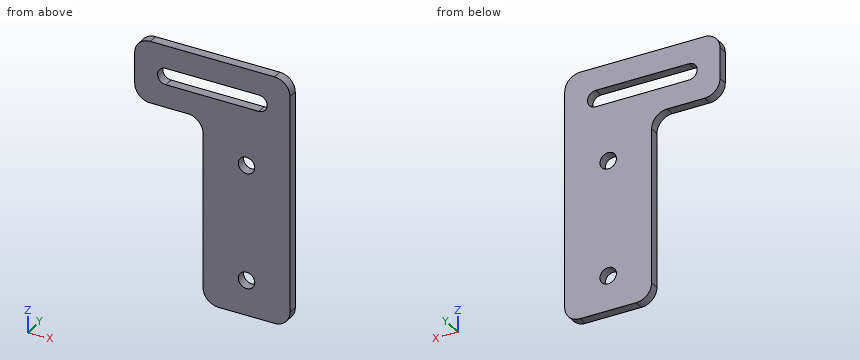
Autodesk Inventor part; units mm, degrees
ref_plane "YZ Plane" through (0, 0, 0) normal (1, 0, 0) x (0, 1, 0)
ref_plane "XZ Plane" through (0, 0, 0) normal (0, 1, 0) x (-1, 0, 0)
ref_plane "XY Plane" through (0, 0, 0) normal (0, 0, 1) x (1, 0, 0)
sketch "Sketch1" plane through (0, 0, 0) normal (0, 1, 0) x (-1, 0, 0)
  line L0 (-25, 40) -> (25, 40)
  line L1 (25, 40) -> (25, -40)
  line L2 (25, -40) -> (-25, -40)
  line L3 (-25, -40) -> (-25, 40)
  line L4 (-25, 40) -> (25, -40) construction
  line L5 (25, 40) -> (-25, -40) construction
  point P0 (0, 0)
  dimension "d0" = 50
  dimension "d1" = 80
extrude "Extrusion1" add sketch "Sketch1" along normal blind 3
sketch "Sketch2" plane through (0, 3, 0) normal (0, 1, 0) x (1, 0, 0)
  line L0 (25, -40) -> (25, 40)
  line L1 (25, 40) -> (11, 40)
  line L2 (11, 40) -> (11, 28.65)
  line L3 (11, 28.65) -> (25, 28.65)
  line L4 (25, 28.65) -> (25, 40)
  line L5 (11, 28.65) -> (11, -8.65)
  circle A0 centre (11, 28.65) radius 2.65
  circle A1 centre (11, -8.65) radius 2.65
  line L6 (-25, -40) -> (25, -40)
  line L7 (-25, 40) -> (-25, -40)
  line L8 (25, -40) -> (-25, -40)
  line L9 (-25, -40) -> (-25, -30)
  line L10 (-25, -30) -> (25, -30)
  line L11 (25, -30) -> (25, -40)
  line L12 (25, -30) -> (15, -30)
  line L13 (-25, -30) -> (-15, -30)
  line L14 (-15, -30) -> (15, -30) construction
  line L15 (-15, -32.65) -> (15, -32.65)
  line L16 (15, -27.35) -> (-15, -27.35)
  arc A2 (-15, -27.35) -> (-15, -32.65) centre (-15, -30) ccw
  arc A3 (15, -32.65) -> (15, -27.35) centre (15, -30) ccw
  line L17 (-25, -30) -> (-25, 40)
  line L18 (-25, 40) -> (-3, 40)
  line L19 (-3, 40) -> (-3, -20)
  line L20 (-3, -20) -> (-25, -20)
  point P0 (0, 0)
  point P1 (0, -30)
  dimension "d4" = 14
  dimension "d5" = 11.35
  dimension "d6" = 37.3
  dimension "d7" = 5.3
  dimension "d8" = 5.3
  dimension "d9" = 10
  dimension "d10" = 10
  dimension "d11" = 10
  dimension "d12" = 5.3
  dimension "d13" = 22
  dimension "d14" = 60
extrude "Extrusion2" cut sketch "Sketch2" against normal through all contours L7 L18 L19 L20 | A1 | A3 L15 A2 L10 | L10 A2 L16 A3 | A0 L5 L3 | L3 L2 A0 | L5 A0 L2
fillet "Fillet1" radius 5 6 edges at (-25, 1.5, 40) (25, 1.5, 40) (25, 1.5, -40) (-3, 1.5, -40) (-3, 1.5, 20) (-25, 1.5, 20)
properties part number "LeadScrewEndMount"
Verification items for the finished model (mm, model axes). Round coordinates to 2 decimals unless told otherwise and drop trailing zeros. Write each loop counter-clockwise with the first axis right and the second up, starting at its lowest first coordinate (ties: lowest second). Pieces come first, ordered by that corner, then holes.
1. Section check C-C on y = 2. Enter the section's corners in (x, z), plus the area to 3 significant figures.
2. Section check A-A on x = 11. Enter the section's corners in (y, z), plus the area to 3 significant figures.
3. Scan lines: L1, parallel to Z at x = 11, y = 0.95; L2, parallel to X at y = 1.8, z = -28.65; L3, parallel to X at y = 2.8, z = -23.5. Record each from-to range of solid material in increasing order.
4. Section check D-D on x = 16. Enter the section's corners in (y, z), plus the area to 3 significant figures.
5. Gauge pin test, flat ends, axial feed: P1, Ø1.5, axis at y = 1, z = -6.5, coming from the -X side; P2, Ø3, axis at x = 11, z = 8.65, coming from the +Y side. Record the tip position at first contact, or that the pin passes through.
6. Section check B-B on z = -28.65. Enter the section's corners in (x, y), plus the area to 3 significant figures.
Answer:
1. outline: (-25, 25) arc R5 ccw to (-20, 20) - (-8, 20) arc R5 cw to (-3, 15) - (-3, -35) arc R5 ccw to (2, -40) - (20, -40) arc R5 ccw to (25, -35) - (25, 35) arc R5 ccw to (20, 40) - (-20, 40) arc R5 ccw to (-25, 35) - close; hole (-15, 27.35) - (15, 27.35) arc R2.65 ccw to (15, 32.65) - (-15, 32.65) arc R2.65 ccw to start; hole circle Ø5.3 at (11, -28.65); hole circle Ø5.3 at (11, 8.65)
1. area: 2,430 mm2
2. outline: (0, -40) - (3, -40) - (3, -31.3) - (0, -31.3) - close; (0, -26) - (3, -26) - (3, 6) - (0, 6) - close; (0, 11.3) - (3, 11.3) - (3, 27.35) - (0, 27.35) - close; (0, 32.65) - (3, 32.65) - (3, 40) - (0, 40) - close
2. area: 192 mm2
3. L1: z = -40 to -31.3, -26 to 6, 11.3 to 27.35, 32.65 to 40
3. L2: x = -3 to 8.35, 13.65 to 25
3. L3: x = -3 to 25
4. outline: (0, -40) - (3, -40) - (3, 27.55) - (0, 27.55) - close; (0, 32.45) - (3, 32.45) - (3, 40) - (0, 40) - close
4. area: 225 mm2
5. P1: stops at x = -3
5. P2: passes through
6. outline: (-3, 0) - (8.35, 0) - (8.35, 3) - (-3, 3) - close; (13.65, 0) - (25, 0) - (25, 3) - (13.65, 3) - close
6. area: 68.1 mm2
